```python
from build123d import *

# Parameters (mm, degrees)
SKETCH001_R  = 15.261185
POCKET_DEPTH = 14


with BuildPart() as part:
    # Sketch (on DatumPlane) → Revolution (revolve)
    with BuildSketch(Plane.XZ):
        Polygon((30, 6), (0.75, 56.662486), (0, 56.662486), (0, 48.662486), (22, 10.557368), (22, 0), (26, 0), (26, 2), align=None)
    revolve(axis=Axis((0, 0, 0), (0, 0, 1)))

    # Sketch001 (on DatumPlane) → Pocket (cut)
    with BuildSketch(Plane.XY.offset(45)):
        Circle(SKETCH001_R)
    extrude(amount=POCKET_DEPTH, mode=Mode.SUBTRACT)


solid = part.part
```
Here's how the part is built. I have some questions about the finished solid (model axes, mm). A direction names the side the tool comes from. Give positions to 0.01 mm unless a question says otherwise; leave off trailing zeros. Loops run counter-clockwise (first coordinate to the right, second up) from the corner with the lowest first, then second, coordinate; pieces in that order, holes last. Notation, with made-up numbers: M -4,0 L 31,0 A8 ccw 31,6 Z; hole C 12.5,69.25 d1. An arc over 180 degrees is marked long. Use one line per item in the form item = value. Start each with the question number.
Q1. If we section it at A-A (y = 0): Write out the boundary of the cut face in (x, z).
Q2. I need wall thicknesses on line 1 along X through (y, z) = (-11, 18); line 2 along Y through (x, z) = (0, 7); line 3 along X through (y, z) = (18.5, 6.5). Which ranges of each line are inside material? Lowest first, please.
Q3. If we section it at D-D (z = 14): Write out the boundary of the cut face in (x, y), then the cut area to 3 significant figures.
Q4. Thinking about a two-plate mould opening in Y: for faces 3 (the conical face through (4.61, -8.86, 31.36)), 4 (the cylindrical face through (-4.769, -21.477, 5.205)), 5 (the conical face through (-26.225, 1.154, 2.25)), 6 (the flat face through (19, 12, 0)), which applies, +Y half, -Y half, draft (parallel to the pull), parting line (faces both ways), or undercut?
Q5. If we section it at C-C (z = 22): Write out the boundary of the cut face in (x, y), then the cut area to 3 significant figures.
Q6. Which directions (+Z, -Z, +X, -X, +Y, -Y) give clear straight access to the entire face, cutting with the end or side of a thin tool? Please do faces 1 (the flat face through (2, -2, 45)), 2 (the cylindrical face through (-20.633, -15.821, 1.014)).
Q7. Will these pins go through, and if not, where does the flat tip stop? pin 1 Ø6 at (y, z) = (12.5, 15) entering from +X; pin 2 Ø1 at (y, z) = (-19.5, 8) entering from -X; pin 3 Ø8 at (x, y) = (9.5, 10) entering from +Z.
Taken from the geometry:
q1.outline = M -30,6 L -26,2 L -26,0 L -22,0 L -22,10.56 L -2.11,45 L -7.48,45 Z; M 2.11,45 L 22,10.56 L 22,0 L 26,0 L 26,2 L 30,6 L 7.48,45 Z
q2.line_1 = -20.28 to -13.87, 13.87 to 20.28
q2.line_2 = -29.42 to -22, 22 to 29.42
q2.line_3 = -23.25 to -11.91, 11.91 to 23.25
q3.outline = C 0,0 d50.76; hole C 0,0 d40.02
q3.area = 766 mm^2
q4.face_3 = undercut
q4.face_4 = undercut
q4.face_5 = parting line
q4.face_6 = draft
q5.outline = C 0,0 d41.52; hole C 0,0 d30.79
q5.area = 610 mm^2
q6.face_1 = +Z, +X, -X, +Y, -Y
q6.face_2 = -Z
q7.pin_1 = 23.9
q7.pin_2 = -21.85
q7.pin_3 = 41
